The listing builds one solid part. Answer for the finished solid, in the listing's coordinates (mm). Face numbers are marked on the shaded views. A direction names the side the tool comes from. Give positions to 0.01 mm unless a question says otherwise; leave off trailing zeros. Write each loop counter-clockwise with the first axis right and the second up, starting at its lowest first coordinate (ties: lowest second). Pieces come first, ordered by that corner, then holes. Notation, with made-up numbers: (79.5, 53.25) - (85.5, 53.25) arc R23 cw to (85.5, 81.25) - close; hole circle Ø1 at (45.5, -17.5). An arc over 180 degrees is marked (long way). One line per item, written item: value. Start each with the question number.
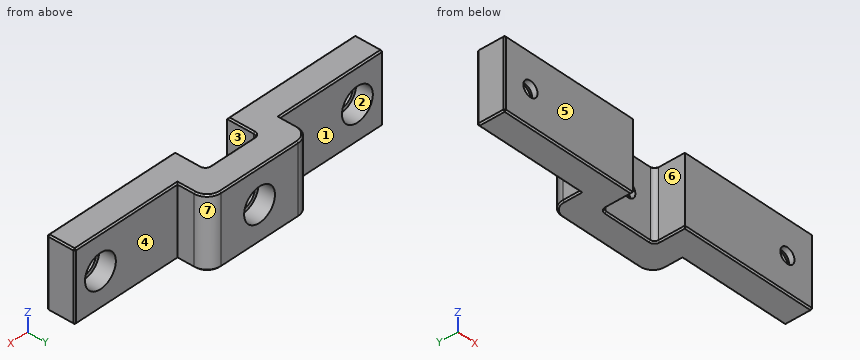
from build123d import *

# Parameters (mm, degrees)
SKETCH1_W               = 120
SKETCH1_H               = 25
BOSS_EXTRUDE1_DEPTH     = 10
SKETCH2_W               = 40
SKETCH2_H               = 25
BOSS_EXTRUDE2_DEPTH     = 11
SKETCH3_W               = 20.2
SKETCH3_H               = 25
CUT_EXTRUDE1_DEPTH      = 11
CUT_EXTRUDE2_DEPTH      = 63.267567802
CUT_EXTRUDE2_DEPTH_BACK = 63.267567802
SKETCH4_R               = 2.75
FILLET1_R               = 5
FILLET2_R               = 1.5
CHAMFER1_SIZE           = 0.5
SKETCH5_R               = 6
CUT_EXTRUDE3_DEPTH      = 6
CHAMFER2_SIZE           = 2
SKETCH6_R               = 6
CUT_EXTRUDE4_DEPTH      = 6
CHAMFER3_SIZE           = 2


with BuildPart() as part:
    # Sketch1 → Boss-Extrude1 (new body)
    with BuildSketch(Plane(origin=(0, 0, 0), x_dir=(1, 0, 0), z_dir=(0, 1, 0))):
        Rectangle(SKETCH1_W, SKETCH1_H)
    extrude(amount=BOSS_EXTRUDE1_DEPTH)

    # Sketch2 → Boss-Extrude2 (add)
    with BuildSketch(Plane(origin=(0, 10, 0), x_dir=(1, 0, 0), z_dir=(0, 1, 0))):
        Rectangle(SKETCH2_W, SKETCH2_H)
    extrude(amount=BOSS_EXTRUDE2_DEPTH)

    # Sketch3 → Cut-Extrude1 (cut)
    with BuildSketch(Plane(origin=(0, 0, 0), x_dir=(1, 0, 0), z_dir=(0, 1, 0))):
        Rectangle(SKETCH3_W, SKETCH3_H)
    extrude(amount=CUT_EXTRUDE1_DEPTH, mode=Mode.SUBTRACT)

    # Sketch4 → Cut-Extrude2 (cut, two sides: drawn at the far end of the back side and taken through both)
    with BuildSketch(Plane.XZ.offset(-11).offset(-CUT_EXTRUDE2_DEPTH_BACK)):
        with Locations(Location((0, 0, 0), (0, 0, 270))):
            Circle(SKETCH4_R)
        with Locations(Location((-50, 0, 0), (0, 0, 270))):
            Circle(SKETCH4_R)
        with Locations(Location((50, 0, 0), (0, 0, 270))):
            Circle(SKETCH4_R)
    extrude(amount=CUT_EXTRUDE2_DEPTH + CUT_EXTRUDE2_DEPTH_BACK, mode=Mode.SUBTRACT)

    # Fillet1
    fillet1_edges = [part.edges().sort_by_distance(p)[0] for p in [
        (-20, 21, 0),
        (20, 21, 0),
    ]]
    fillet(fillet1_edges, radius=FILLET1_R)

    # Fillet2
    fillet2_edges = [part.edges().sort_by_distance(p)[0] for p in [
        (-10.1, 11, 0),
        (10.1, 11, 0),
    ]]
    fillet(fillet2_edges, radius=FILLET2_R)

    # Chamfer1
    chamfer1_edges = [part.edges().sort_by_distance(p)[0] for p in [
        (60, 10, 0),
        (40, 10, 12.5),
        (-40, 10, -12.5),
        (40, 10, -12.5),
        (-35.05, 0, -12.5),
        (35.05, 0, 12.5),
        (-60, 10, 0),
        (35.05, 0, -12.5),
        (60, 0, 0),
        (-35.05, 0, 12.5),
        (0, 21, 12.5),
        (0, 21, -12.5),
        (20, 13, 12.5),
        (-20, 13, 12.5),
        (18.535533906, 19.535533906, 12.5),
        (-60, 0, 0),
        (-18.535533906, 19.535533906, 12.5),
        (-20, 13, -12.5),
        (20, 13, -12.5),
        (18.535533906, 19.535533906, -12.5),
        (-18.535533906, 19.535533906, -12.5),
        (10.1, 4.75, 12.5),
        (10.1, 4.75, -12.5),
        (0, 11, -12.5),
        (0, 11, 12.5),
        (-10.1, 4.75, -12.5),
        (-10.1, 4.75, 12.5),
        (9.660660172, 10.560660172, -12.5),
        (9.660660172, 10.560660172, 12.5),
        (-9.660660172, 10.560660172, 12.5),
        (-9.660660172, 10.560660172, -12.5),
        (-60, 5, -12.5),
        (60, 5, -12.5),
        (60, 5, 12.5),
        (-60, 5, 12.5),
        (-40, 10, 12.5),
    ]]
    chamfer(chamfer1_edges, length=CHAMFER1_SIZE)

    # Sketch5 → Cut-Extrude3 (cut)
    with BuildSketch(Plane(origin=(0, 10, 0), x_dir=(1, 0, 0), z_dir=(0, 1, 0))):
        with Locations(Location((-50, 0, 0), (0, 0, 270))):
            Circle(SKETCH5_R)
        with Locations(Location((50, 0, 0), (0, 0, 270))):
            Circle(SKETCH5_R)
    extrude(amount=-CUT_EXTRUDE3_DEPTH, mode=Mode.SUBTRACT)

    # Chamfer2
    chamfer2_edges = [part.edges().sort_by_distance(p)[0] for p in [
        (-50, 4, 2.75),
        (50, 4, 2.75),
    ]]
    chamfer(chamfer2_edges, length=CHAMFER2_SIZE)

    # Sketch6 → Cut-Extrude4 (cut)
    with BuildSketch(Plane(origin=(0, 21, 0), x_dir=(1, 0, 0), z_dir=(0, 1, 0))):
        with Locations(Location((0, 0, 0), (0, 0, 270))):
            Circle(SKETCH6_R)
    extrude(amount=-CUT_EXTRUDE4_DEPTH, mode=Mode.SUBTRACT)

    # Chamfer3
    chamfer3_edges = [part.edges().sort_by_distance(p)[0] for p in [
        (0, 15, 2.75),
    ]]
    chamfer(chamfer3_edges, length=CHAMFER3_SIZE)


solid = part.part
Item 1: Find section B-B on x = 0. Determine the outline of the cut face in (y, z).
Item 2: Straight lines are drawn through the part: line 1 along X through (y, z) = (1, 0); line 2 along X through (y, z) = (6.6, 0); line 3 along Z through (x, y) = (0, 11.6). For each, find the intervals that lie inside material, in ascending order.
Item 3: The mould has two halves that part along Y. Classify the marked faces 5, 6 and 7: +Y half, -Y half, draft (parallel to the pull), parting line (faces both ways), or undercut.
Item 4: Find section C-C on y = 8. Determine the outline of the cut face in (x, z).
Item 5: Find section D-D on x = -41.5. Determine the outline of the cut face in (y, z), plus the area to 4 significant figures.
Item 6: Find section A-A on y = 3. Determine the outline of the cut face in (x, z).
Item 7: Each of these flat-tipped pins is pushed along its axis until it touches: pin 1 Ø10 at (y, z) = (11.5, -1) entering from -X; pin 2 Ø1 at (x, z) = (-5, -0.5) entering from -Y; pin 3 Ø3 at (y, z) = (13, 2) entering from +X; pin 4 Ø2 at (x, z) = (36, -3) entering from +Y. Where does it stop, or does it pass through?
Item 8: For the marked faces 1, 2, 3 and 4, determine the directions among +Z, -Z, +X, -X, +Y, -Y from which every point of the face is accessible in a straight line to the end or side of a thin tool.
Values:
1. outline: (11, -12) - (11.5, -12.5) - (20.5, -12.5) - (21, -12) - (21, -6) - (15, -6) - (15, -4.75) - (13, -2.75) - (11, -2.75) - close; (11, 2.75) - (13, 2.75) - (15, 4.75) - (15, 6) - (21, 6) - (21, 12) - (20.5, 12.5) - (11.5, 12.5) - (11, 12) - close
2. line 1: -60 to -52.75, -47.25 to -10.1, 10.1 to 47.25, 52.75 to 60
2. line 2: -60 to -56, -44 to -10.1, 10.1 to 44, 56 to 60
2. line 3: -12.5 to -2.75, 2.75 to 12.5
3. face 5: -Y half
3. face 6: draft
3. face 7: +Y half
4. outline: (-60, -12) - (-59.5, -12.5) - (-10.6, -12.5) - (-10.1, -12) - (-10.1, 12) - (-10.6, 12.5) - (-59.5, 12.5) - (-60, 12) - close; (10.1, -12) - (10.6, -12.5) - (59.5, -12.5) - (60, -12) - (60, 12) - (59.5, 12.5) - (10.6, 12.5) - (10.1, 12) - close; hole circle Ø12 at (-50, 0); hole circle Ø12 at (50, 0)
5. outline: (0, -12) - (0.5, -12.5) - (9.5, -12.5) - (10, -12) - (10, 12) - (9.5, 12.5) - (0.5, 12.5) - (0, 12) - close
5. area: 249.5 mm^2
6. outline: (-60, -12) - (-59.5, -12.5) - (-10.6, -12.5) - (-10.1, -12) - (-10.1, 12) - (-10.6, 12.5) - (-59.5, 12.5) - (-60, 12) - close; (10.1, -12) - (10.6, -12.5) - (59.5, -12.5) - (60, -12) - (60, 12) - (59.5, 12.5) - (10.6, 12.5) - (10.1, 12) - close; hole circle Ø7.5 at (-50, 0); hole circle Ø7.5 at (50, 0)
7. pin 1: x = -60
7. pin 2: y = 11
7. pin 3: x = 20
7. pin 4: y = 10
8. face 1: +Z, -Z, -X, +Y
8. face 2: +Y
8. face 3: +Z, -Z, -Y
8. face 4: +Z, -Z, +X, +Y
